Source: CAD feature listing. Evaluate the final solid. Frame: model axes, mm. Face numbers are marked on the shaded views. A direction names the side the tool comes from. Round coordinates to 2 decimals unless told otherwise and drop trailing zeros. Loops run counter-clockwise (first coordinate to the right, second up) from the corner with the lowest first, then second, coordinate; pieces in that order, holes last. Notation, with made-up numbers: M 24.25,27 L 66.25,27 A29 cw 66.25,49 Z; hole C -5.75,33.5 d1. An arc over 180 degrees is marked long. Answer as a JSON object with one key per item and string values.
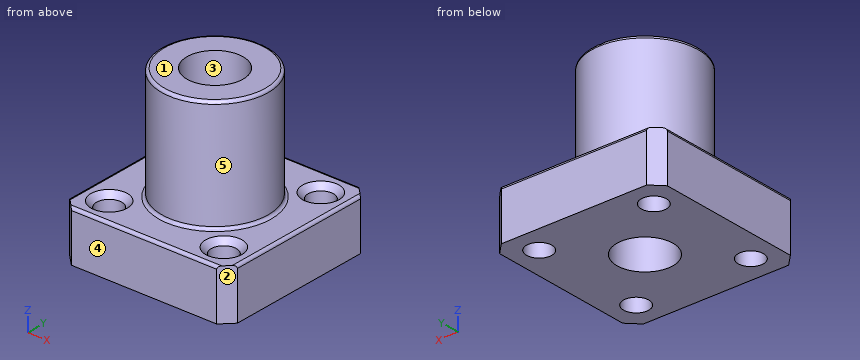
from build123d import *

# Parameters (mm, degrees)
SKETCH1_W                    = 30
SKETCH1_H                    = 30
BOSS_EXTRUDE1_DEPTH          = 9
SKETCH2_R                    = 9.5
BOSS_EXTRUDE2_DEPTH          = 20
SKETCH3_R                    = 5
CUT_EXTRUDE1_DEPTH           = 36.930488446
SKETCH4_R                    = 2.25
CUT_EXTRUDE2_DEPTH           = 36.930488446
CHAMFER1_SIZE                = 1
CIRPATTERN1_COUNT            = 4
CHAMFER1_OF_CIRPATTERN1_SIZE = 1
FILLET1_R                    = 0.5
CHAMFER2_SIZE                = 2


with BuildPart() as part:
    # Sketch1 → Boss-Extrude1 (new body)
    with BuildSketch(Plane.XY):
        Rectangle(SKETCH1_W, SKETCH1_H)
    extrude(amount=BOSS_EXTRUDE1_DEPTH)

    # Sketch2 → Boss-Extrude2 (add)
    with BuildSketch(Plane.XY.offset(9)):
        Circle(SKETCH2_R)
    extrude(amount=BOSS_EXTRUDE2_DEPTH)

    # Sketch3 → Cut-Extrude1 (cut, through all)
    with BuildSketch(Plane.XY.offset(29)):
        Circle(SKETCH3_R)
    extrude(amount=-CUT_EXTRUDE1_DEPTH, mode=Mode.SUBTRACT)

    # Sketch4 → Cut-Extrude2 (cut, through all)
    with BuildSketch(Plane(origin=(0, 0, 0), x_dir=(-1, 0, 0), z_dir=(0, 0, -1))):
        with Locations((-10.253048327, 10.253048327)):
            Circle(SKETCH4_R)
    cut_extrude2 = extrude(amount=-CUT_EXTRUDE2_DEPTH, mode=Mode.SUBTRACT)

    # Chamfer1
    chamfer1_edges = [part.edges().sort_by_distance(p)[0] for p in [
        (12.503048327, 10.253048327, 9),
    ]]
    chamfer(chamfer1_edges, length=CHAMFER1_SIZE)

    # CirPattern1: Cut-Extrude2 ×4 about axis
    cirpattern1_axis = Axis((0, 0, 0), (0, 0, 1))
    for i in range(1, CIRPATTERN1_COUNT):
        add(cut_extrude2.rotate(cirpattern1_axis, i * 360 / CIRPATTERN1_COUNT), mode=Mode.SUBTRACT)

    # Chamfer1 of CirPattern1
    chamfer1_of_cirpattern1_edges = [part.edges().sort_by_distance(p)[0] for p in [
        (-10.253048327, 12.503048327, 9),
        (-12.503048327, -10.253048327, 9),
        (10.253048327, -12.503048327, 9),
    ]]
    chamfer(chamfer1_of_cirpattern1_edges, length=CHAMFER1_OF_CIRPATTERN1_SIZE)

    # Fillet1
    fillet1_edges = [part.edges().sort_by_distance(p)[0] for p in [
        (-15, 0, 9),
        (0, -15, 9),
        (-9.5, 0, 9),
        (-9.5, 0, 29),
        (15, 0, 9),
        (0, 15, 9),
    ]]
    fillet(fillet1_edges, radius=FILLET1_R)

    # Chamfer2
    # the kernel refuses this chamfer: 2 mm, written as the material it takes off along each edge
    with BuildSketch(Plane(origin=(15, -15, -5.143365976), x_dir=(-0.9996219169112968, -0.027495876610586487, 0), z_dir=(0, 0, 1)), Plane(origin=(-15, -15, -5.143365976), x_dir=(-0.027495876610586487, 0.9996219169112968, 0), z_dir=(0, 0, 1))) as chamfer2_piece_1:
        Polygon((CHAMFER2_SIZE * 0.999621916911, -CHAMFER2_SIZE * 0.0274958766106), (-CHAMFER2_SIZE * 0.0274958766106, -CHAMFER2_SIZE * 0.999621916911), (0, 0), align=None)
    extrude(amount=18.786731952, mode=Mode.SUBTRACT)
    with BuildSketch(Plane(origin=(15, 15, -5.143365976), x_dir=(-0.9996219169112968, 0.027495876610586487, 0), z_dir=(0, 0, 1)), Plane(origin=(-15, 15, -5.143365976), x_dir=(-0.027495876610586487, -0.9996219169112968, 0), z_dir=(0, 0, 1))) as chamfer2_piece_2:
        Polygon((CHAMFER2_SIZE * 0.999621916911, CHAMFER2_SIZE * 0.0274958766106), (-CHAMFER2_SIZE * 0.0274958766106, CHAMFER2_SIZE * 0.999621916911), (0, 0), align=None)
    extrude(amount=18.786731952, mode=Mode.SUBTRACT)


solid = part.part
Item 1: Section A-A on y = 0. Return the cut outline in (x, z), then the cut area to 3 significant figures.
Answer sheet:
{"outline": "M -15,0 L -5,0 L -5,29 L -9,29 A0.5 ccw -9.5,28.5 L -9.5,9.5 A0.5 cw -10,9 L -14.5,9 A0.5 ccw -15,8.5 Z; M 5,0 L 15,0 L 15,8.5 A0.5 ccw 14.5,9 L 10,9 A0.5 cw 9.5,9.5 L 9.5,28.5 A0.5 ccw 9,29 L 5,29 Z", "area": "360 mm²"}
Item 2: Access query for the marked faces 4 and 5. Directions: +Z, -Z, +X, -X, +Y, -Y. A direction counts if a zero-diameter tool reaches every point of the face in a straight line with its end or side. Return the directions, or none.
Answer sheet:
{"face 4": "+Z, -Z, +X, -X, -Y", "face 5": "+Z"}
Item 3: Section C-C on z = 27. Return the cut outline in (x, y).
Answer sheet:
{"outline": "C 0,0 d19; hole C 0,0 d10"}
Item 4: Pull-direction query (Y, two-part tool) for the marked faces 1, 2 and 3; classes: pulls with the +Y half, pulls with the -Y half, needs draft (parallel to the pull), parting line crosses it, or undercut.
Answer sheet:
{"face 1": "needs draft", "face 2": "pulls with the -Y half", "face 3": "undercut"}
Item 5: Section D-D on z = 5. Return the cut outline in (x, y).
Answer sheet:
{"outline": "M -15,-13 L -13,-15 L 13,-15 L 15,-13 L 15,13 L 13,15 L -13,15 L -15,13 Z; hole C -10.25,-10.25 d4.5; hole C -10.25,10.25 d4.5; hole C 0,0 d10; hole C 10.25,-10.25 d4.5; hole C 10.25,10.25 d4.5"}
Item 6: Line query: probe 1 along Z at (x, y) = (-3, -12.5); probe 2 along Y at (x, z) = (3.5, 10); probe 3 along X at (y, z) = (1.5, 3.5). Output: solid intervals per line, ascending. Write a range as from..to.
Answer sheet:
{"probe 1": "z = 0..9", "probe 2": "y = -8.83..-3.57, 3.57..8.83", "probe 3": "x = -15..-4.77, 4.77..15"}
Item 7: Contact query for flat-ended pins moving along their axis: pin 1 Ø10 at (y, z) = (-6, 24) entering from -X; pin 2 Ø3 at (x, y) = (8.5, 11) entering from +Z. Output: stop coordinate, or through.
Answer sheet:
{"pin 1": "stops at x = -9.45", "pin 2": "stops at z = 9"}
